The model under review builds one solid part; all positions refer to its coordinate system, in mm. Give positions to 0.01 mm unless a question says otherwise; leave off trailing zeros. Write each loop counter-clockwise with the first axis right and the second up, starting at its lowest first coordinate (ties: lowest second). Pieces come first, ordered by that corner, then holes. Notation, with made-up numbers: M 76,20.5 L 118,20.5 A27 cw 118,38.5 Z; hole C 79,-26.75 d3. An arc over 180 degrees is marked long. Write each question's results on one line, items separated by ' | '. Start each with the question number.
Autodesk Inventor part; units mm, degrees
ref_plane "Work Plane1" through (4.7798, -19.0607, 0) normal (0, 0, 1) x (1, -0.0002116, 0)
ref_plane "YZ Plane" through (0, 0, 0) normal (1, 0, 0) x (0, 1, 0)
ref_plane "XZ Plane" through (0, 0, 0) normal (0, 1, 0) x (-1, 0, 0)
ref_plane "Work Plane1" through (4.7798, -19.0607, 0) normal (0, 0, 1) x (1, -0.0002116, 0)
sketch "Sketch1" plane through (4.7798, -19.0607, 0) normal (0, 0, 1) x (1, -0.0002116, 0)
  circle A0 centre (-10.4, -140.7495) radius 4.3281
  arc A1 (-17.3999, -140.717) -> (-3.4, -140.7495) centre (-10.4, -140.7495) ccw
  arc A2 (2, 1237.5744) -> (-10.9999, 1237.6046) centre (-4.5, 1237.5744) ccw
  line L0 (-17.3999, -140.717) -> (-10.9999, 1237.6046)
  line L1 (-3.4, -140.7495) -> (-3.4, 11.2032)
  line L2 (2, 1237.5744) -> (2, 37.9844)
  line L3 (0.5, 37.9844) -> (0.5, 1237.5744)
  arc A3 (0.5, 1237.5744) -> (-9.4999, 1237.5976) centre (-4.5, 1237.5744) ccw
  line L4 (-9.4999, 1237.5976) -> (-15.8999, -140.724)
  line L5 (-4.9, 11.2032) -> (-4.9, -140.7495)
  arc A4 (-15.8999, -140.724) -> (-4.9, -140.7495) centre (-10.4, -140.7495) ccw
  line L6 (-4.9, 11.2032) -> (-3.4, 11.2032)
  line L7 (0.5, 37.9844) -> (2, 37.9844)
  point P0 (-4.7838, 19.0597)
  dimension "d3" = 1.5
  dimension "d4" = 1.5
  dimension "d5" = 5.5
  dimension "d6" = 5
extrude "Extrusion1" add sketch "Sketch1" along normal mid plane 6 contours L0 A2 L2 L7 L3 A3 L4 A4 L5 L6 L1 A1
properties part number "FDM20-BandaX-01"
(1) Clearance check with flat-ended pins moving along their axes: P1, Ø1, axis at x = -3, z = -0.5, coming from the +Y side; P2, Ø1.8, axis at y = -96.5, z = -0.5, coming from the -X side; P3, Ø1.5, axis at y = 516.5, z = -1, coming from the -X side. State where each tip first meets the part, or that it passes through.
(2) Wall thickness on L1, parallel to X at y = 874, z = 0.8; L2, parallel to Y at x = -1.75, z = 2.3; L3, parallel to X at y = 864, z = 0: over which ranges is each line inside the solid? List them lowest first.
(3) Add section B-B (z = -1.8). State the section outline as (x, y) points, then the cut area to 3 significant figures.
(4) Add section A-A (y = 316.5). State the section outline as (x, z) points.
Calculated:
1) P1: stops at y = 1224.26 | P2: stops at x = -12.35 | P3: stops at x = -9.37
2) L1: x = -7.63 to -6.13, 5.47 to 6.97 | L2: y = -165.62 to -163.69, 1222.96 to 1224.6 | L3: x = -7.68 to -6.18, 5.47 to 6.97
3) outline: M -12.65,-159.77 A7 ccw 1.35,-159.81 L 1.38,-7.86 L -0.12,-7.86 L -0.15,-159.81 A5.5 cw -11.15,-159.78 L -4.46,1218.54 A5 cw 5.54,1218.51 L 5.29,18.92 L 6.79,18.92 L 7.04,1218.51 A6.5 ccw -5.96,1218.55 Z | area: 4,150 mm²
4) outline: M -10.34,-3 L -8.84,-3 L -8.84,3 L -10.34,3 Z; M 5.35,-3 L 6.85,-3 L 6.85,3 L 5.35,3 Z
